```python
from build123d import *

# Parameters (mm, degrees)
SKETCH1_W           = 70
SKETCH1_H           = 24
BOSS_EXTRUDE1_DEPTH = 2
SKETCH2_W           = 20
SKETCH2_H           = 4
BOSS_EXTRUDE2_DEPTH = 30
FILLET1_R           = 10
FILLET2_R           = 10
CUT_EXTRUDE1_REACH  = 55.151
SKETCH3_R           = 1.5
FILLET3_R           = 10
SKETCH4_R           = 2.05
CUT_EXTRUDE2_DEPTH  = 4
SKETCH5_R           = 3
CUT_EXTRUDE3_DEPTH  = 2.5
CUT_EXTRUDE4_DEPTH  = 2.5


with BuildPart() as part:
    # Sketch1 → Boss-Extrude1 (new, symmetric)
    with BuildSketch(Plane(origin=(0, 0, 0), x_dir=(1, 0, 0), z_dir=(0, 1, 0))):
        Rectangle(SKETCH1_W, SKETCH1_H)
    extrude(amount=BOSS_EXTRUDE1_DEPTH, both=True)

    # Sketch2 → Boss-Extrude2 (add)
    with BuildSketch(Plane(origin=(0, 2, 0), x_dir=(1, 0, 0), z_dir=(0, 1, 0))):
        with Locations((0, 10)):
            Rectangle(SKETCH2_W, SKETCH2_H)
        with Locations((0, -10)):
            Rectangle(SKETCH2_W, SKETCH2_H)
    extrude(amount=BOSS_EXTRUDE2_DEPTH)

    # Fillet1
    fillet1_edges = [part.edges().sort_by_distance(p)[0] for p in [
        (-10, 2, -10),
        (10, 2, -10),
        (-10, 2, 10),
        (10, 2, 10),
    ]]
    fillet(fillet1_edges, radius=FILLET1_R)

    # Fillet2
    fillet2_edges = [part.edges().sort_by_distance(p)[0] for p in [
        (-10, 32, 10),
        (10, 32, 10),
        (10, 32, -10),
        (-10, 32, -10),
    ]]
    fillet(fillet2_edges, radius=FILLET2_R - 0.0001)  # a hair under: the kernel refuses the full size

    # Cut-Extrude1: up to this face of the body (flat: up to its plane)
    cut_extrude1_end = Plane(part.part.faces().sort_by_distance((0, 10.345619741, -12))[0])
    # Sketch3 → Cut-Extrude1 (cut, up to the picked face)
    with BuildSketch(Plane.XY.offset(12), mode=Mode.PRIVATE) as cut_extrude1_sk1:
        with Locations((0, 24)):
            Circle(SKETCH3_R)
    cut_extrude1_tool1 = split(extrude(cut_extrude1_sk1.sketch, amount=-CUT_EXTRUDE1_REACH, mode=Mode.PRIVATE), bisect_by=cut_extrude1_end, keep=Keep.BOTH, mode=Mode.PRIVATE)
    add(cut_extrude1_tool1.solids().sort_by(Axis((0, 24, 12), (0, 0, -1)))[0], mode=Mode.SUBTRACT)

    # Fillet3
    fillet3_edges = [part.edges().sort_by_distance(p)[0] for p in [
        (35, 0, 12),
        (-35, 0, 12),
        (-35, 0, -12),
        (35, 0, -12),
    ]]
    fillet(fillet3_edges, radius=FILLET3_R)

    # Sketch4 → Cut-Extrude2 (cut)
    with BuildSketch(Plane(origin=(0, 2, 0), x_dir=(1, 0, 0), z_dir=(0, 1, 0))):
        with Locations(Location((-26, 0, 0), (0, 0, 270))):
            Circle(SKETCH4_R)
        with Locations(Location((26.78915656, 0, 0), (0, 0, 270))):
            Circle(SKETCH4_R)
    extrude(amount=-CUT_EXTRUDE2_DEPTH, mode=Mode.SUBTRACT)

    # Sketch5 → Cut-Extrude3 (cut)
    with BuildSketch(Plane.XY.offset(12)):
        with Locations((0, 24)):
            Circle(SKETCH5_R)
    extrude(amount=-CUT_EXTRUDE3_DEPTH, mode=Mode.SUBTRACT)

    # Sketch6 → Cut-Extrude4 (cut)
    with BuildSketch(Plane(origin=(0, 0, -12), x_dir=(-1, 0, 0), z_dir=(0, 0, -1))):
        Polygon((2.75, 25.58771324), (0, 27.175426481), (-2.75, 25.58771324), (-2.75, 22.41228676), (0, 20.824573519), (2.75, 22.41228676), align=None)
    extrude(amount=-CUT_EXTRUDE4_DEPTH, mode=Mode.SUBTRACT)


solid = part.part
```
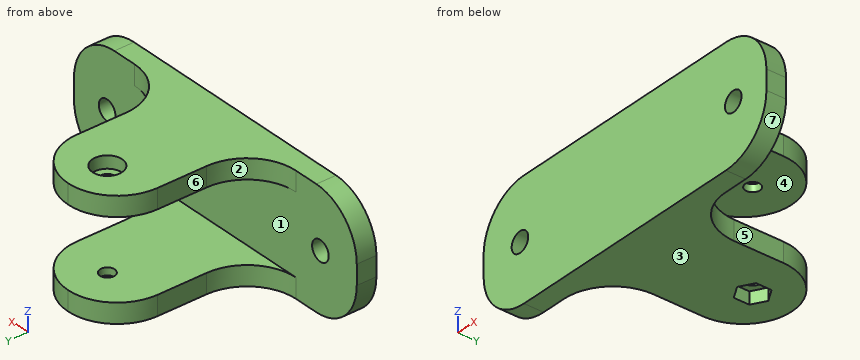
Could you check a few things on this model? Use its own coordinates, in mm. Face numbers are marked on the shaded views. A direction names the side the tool comes from. Give positions to 0.01 mm unless a question says otherwise; leave off trailing zeros. Loops run counter-clockwise (first coordinate to the right, second up) from the corner with the lowest first, then second, coordinate; pieces in that order, holes last. Notation, with made-up numbers: (26.5, -18.5) - (74.5, -18.5) arc R34 cw to (74.5, 17.5) - close; hole circle Ø4 at (38.5, 32.25). An arc over 180 degrees is marked (long way). Answer in a Markdown table with one row per item. Add a question column.
Q1. If we section it at A-A (x = -26): List the corners of the cut face in (y, z) for me, plus the area to 3 significant figures.
Q2. Please list where these lines run through material, in increasing order: L1, parallel to X at y = -0.35, z = 0; L2, parallel to Z at x = 7, y = 16.5; L3, parallel to Y at x = -11.5, z = 6.5. Write a range as from..to.
Q3. If we section it at C-C (y = 24): List the corners of the cut face in (x, z) for me, plus the area to 3 significant figures.
Q4. For pin 1 (2 mm diameter, centred on y = 23.5, z = -11, fed in from +X); pin 2 (1.5 mm diameter, centred on y = 9, z = -8, fed in from -X); pin 3 (2 mm diameter, centred on y = 15.5, z = 10, fed in from -X), each with a flat end and sliding along its axis, tell me the tip position at first contact or that it passes through.
Q5. We'd pull the mould along Z, two halves only. Please class the marked faces 1, 2, 3 and 4: +Z half, -Z half, draft (parallel to the pull), parting line (faces both ways), or undercut.
Q6. Which directions (+Z, -Z, +X, -X, +Y, -Y) give clear straight access to the entire face, cutting with the end or side of a thin tool? Please do the marked faces 5, 6 and 7.
Q7. If we section it at B-B (z = 0): List the corners of the cut face in (x, y) for me, plus the area to 3 significant figures.
The answers:
| question | item | result |
|---|---|---|
| 1 | outline | (-2, -11.95) - (2, -11.95) - (2, -2.05) - (-2, -2.05) - close; (-2, 2.05) - (2, 2.05) - (2, 11.95) - (-2, 11.95) - close |
| 1 | area | 79.2 mm^2 |
| 2 | L1 | x = -35..-28.05, -23.95..24.74, 28.84..35 |
| 2 | L2 | z = -12..-8, 8..12 |
| 2 | L3 | y = -2..2 |
| 3 | outline | (-9.8, -12) - (-2.75, -12) - (-2.75, -9.5) - (-1.5, -9.5) - (-1.5, -8) - (-9.8, -8) - close; (-9.8, 8) - (-1.5, 8) - (-1.5, 9.5) - (-3, 9.5) - (-3, 12) - (-9.8, 12) - close; (1.5, -9.5) - (2.75, -9.5) - (2.75, -12) - (9.8, -12) - (9.8, -8) - (1.5, -8) - close; (1.5, 8) - (9.8, 8) - (9.8, 12) - (3, 12) - (3, 9.5) - (1.5, 9.5) - close |
| 3 | area | 119 mm^2 |
| 4 | pin 1 | stops at x = 9.99 |
| 4 | pin 2 | stops at x = -10.73 |
| 4 | pin 3 | stops at x = -10 |
| 5 | face 1 | undercut |
| 5 | face 2 | draft |
| 5 | face 3 | -Z half |
| 5 | face 4 | undercut |
| 6 | face 5 | +Z, -Z, +X, +Y |
| 6 | face 6 | +Z, -Z, -X, +Y |
| 6 | face 7 | -Z, +X, +Y, -Y |
| 7 | outline | (-35, -2) - (-28.05, -2) - (-28.05, 2) - (-35, 2) - close; (-23.95, -2) - (24.74, -2) - (24.74, 2) - (-23.95, 2) - close; (28.84, -2) - (35, -2) - (35, 2) - (28.84, 2) - close |
| 7 | area | 247 mm^2 |
